from build123d import *

# Parameters (mm, degrees)
HEX_2_DEPTH = 3.048


with BuildPart() as part:
    # BodySke → Base-Revolve (revolve)
    with BuildSketch(Plane.XY, mode=Mode.PRIVATE) as base_revolve_sk:
        Polygon((0, 0), (0, 4.1275), (0.635, 4.7625), (6.35, 4.7625), (6.35, 3.175), (24.64435, 3.175), (25.4, 2.41935), (25.4, 0), align=None)
    revolve(base_revolve_sk.sketch.rotate(Axis((-31.75, 0, 0), (1, 0, 0)), 90), axis=Axis((-31.75, 0, 0), (1, 0, 0)))

    # Sketch3 → Hex 2 (cut)
    with BuildSketch(Plane(origin=(0, 0, 0), x_dir=(0, 0.500000000000001, 0.866025403784438), z_dir=(-1, 0, 0))):
        Polygon((1.374815329, 2.38125), (-1.374815329, 2.38125), (-2.749630657, 0), (-1.374815329, -2.38125), (1.374815329, -2.38125), (2.749630657, 0), align=None)
    extrude(amount=-HEX_2_DEPTH, mode=Mode.SUBTRACT)


solid = part.part
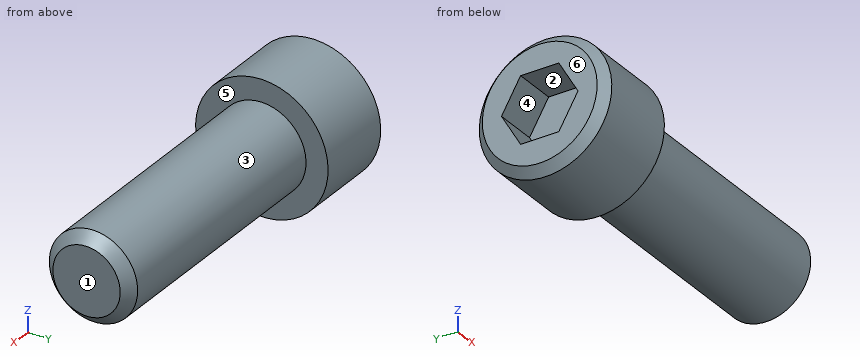
Geometry check sheet. Reference: the model listing, model coordinates, mm. Face numbers are marked on the shaded views. A direction names the side the tool comes from. Give positions to 0.01 mm unless a question says otherwise; leave off trailing zeros. Loops run counter-clockwise (first coordinate to the right, second up) from the corner with the lowest first, then second, coordinate; pieces in that order, holes last.
(1) Set-up check for the marked faces 4, 5 and 6: record each of +Z, -Z, +X, -X, +Y, -Y from which the full face is reachable in a straight line by a thin tool's end or side.
From the geometry:
face 4: -X
face 5: +X
face 6: +Z, -Z, -X, +Y, -Y
(2) Thickness scan on L1, parallel to X at y = 0.25, z = 3.25; L2, parallel to X at y = 0.25, z = -1; L3, parallel to Z at x = 23.75, y = -1. Record the ranges inside material, lowest first.
From the geometry:
L1: x = 0 to 6.35
L2: x = 3.05 to 25.4
L3: z = -3.01 to 3.01
(3) Section check B-B on x = 23. Record the cut outline in (y, z) (3 decimals).
From the geometry:
outline: circle Ø6.35 at (0, 0)
(4) Depth check by flat-ended pin: pin 1 Ø4 at (x, y) = (2.5, -2.5) entering from -Z; pin 2 Ø4 at (x, z) = (12.5, 2.5) entering from -Y; pin 3 Ø3 at (x, z) = (19, 2) entering from +Y. Enter the tip coordinate at first touch or a pass-through.
From the geometry:
pin 1: stops at z = -4.74
pin 2: stops at y = -3.14
pin 3: stops at y = 3.14
(5) Section check C-C on x = 5.25. Record the cut outline in (y, z) (1 decimal), then the cut area to 3 significant figures.
From the geometry:
outline: circle Ø9.5 at (0, 0)
area: 71.3 mm2
(6) Release check for a two-part mould opening along Y. For the marked faces 1, 2 and 3 record: released by +Y, released by -Y, zero draft, split by the parting line, or undercut.
From the geometry:
face 1: zero draft
face 2: undercut
face 3: split by the parting line
